```python
from build123d import *

# Parameters (mm, degrees)
SKETCH6_W                = 42.3
SKETCH6_H                = 42.3
SKETCH6_R                = 1.7
SKETCH6_R_2              = 13.5
BOSS_EXTRUDE4_DEPTH      = 6.35
SKETCH7_W                = 42.3
SKETCH7_H                = 6.35
BOSS_EXTRUDE5_DEPTH      = 6.35
SKETCH9_W                = 6.35
SKETCH9_H                = 6.35
BOSS_EXTRUDE7_DEPTH      = 20
BOSS_EXTRUDE9_DEPTH      = 12.7
BOSS_EXTRUDE9_DEPTH_BACK = 19.05
CUT_EXTRUDE3_DEPTH       = 62.003217128


with BuildPart() as part:
    # Sketch6 → Boss-Extrude4 (new body)
    with BuildSketch(Plane.XY):
        Rectangle(SKETCH6_W, SKETCH6_H)
        with Locations((-15.5, 15.5)):
            Circle(SKETCH6_R, mode=Mode.SUBTRACT)
        with Locations((15.5, 15.5)):
            Circle(SKETCH6_R, mode=Mode.SUBTRACT)
        with Locations((15.5, -15.5)):
            Circle(SKETCH6_R, mode=Mode.SUBTRACT)
        with Locations((-15.5, -15.5)):
            Circle(SKETCH6_R, mode=Mode.SUBTRACT)
        Circle(SKETCH6_R_2, mode=Mode.SUBTRACT)
    extrude(amount=BOSS_EXTRUDE4_DEPTH)

    # Sketch7 → Boss-Extrude5 (add)
    with BuildSketch(Plane(origin=(0, 21.15, 0), x_dir=(1, 0, 0), z_dir=(0, 1, 0))):
        with Locations((0, -3.175)):
            Rectangle(SKETCH7_W, SKETCH7_H)
    extrude(amount=BOSS_EXTRUDE5_DEPTH)

    # Sketch9 → Boss-Extrude7 (add)
    with BuildSketch(Plane(origin=(0, 27.5, 0), x_dir=(1, 0, 0), z_dir=(0, 1, 0))):
        with Locations((-17.975, -3.175)):
            Rectangle(SKETCH9_W, SKETCH9_H)
        with Locations((8.875, -3.175)):
            Rectangle(SKETCH9_W, SKETCH9_H)
    extrude(amount=BOSS_EXTRUDE7_DEPTH)

    # Sketch11 → Boss-Extrude9 (add, two sides: drawn at the far end of the back side and taken through both)
    with BuildSketch(Plane(origin=(0, 0, 0), x_dir=(-1, 0, 0), z_dir=(0, 0, -1)).offset(-BOSS_EXTRUDE9_DEPTH_BACK)):
        Polygon((-12.05, 47.5), (-12.05, 27.5), (-12.05, 21.15), (21.15, 21.15), (21.15, 47.5), (14.8, 47.5), (14.8, 27.5), (-5.7, 27.5), (-5.7, 47.5), align=None)
    extrude(amount=BOSS_EXTRUDE9_DEPTH + BOSS_EXTRUDE9_DEPTH_BACK)

    # Sketch12 → Cut-Extrude3 (cut, through all)
    with BuildSketch(Plane(origin=(12.05, 0, 0), x_dir=(0, 0, -1), z_dir=(1, 0, 0))):
        with BuildLine():
            ThreePointArc((2.5125, 37.5), (4.7625, 35.25), (7.0125, 37.5))
            Line((7.0125, 37.5), (2.5125, 37.5))
        make_face()
        with BuildLine():
            Line((2.5125, 37.5), (7.0125, 37.5))
            ThreePointArc((7.0125, 37.5), (4.7625, 39.75), (2.5125, 37.5))
        make_face()
        with BuildLine():
            ThreePointArc((-13.3625, 37.5), (-11.1125, 35.25), (-8.8625, 37.5))
            Line((-8.8625, 37.5), (-13.3625, 37.5))
        make_face()
        with BuildLine():
            Line((-13.3625, 37.5), (-8.8625, 37.5))
            ThreePointArc((-8.8625, 37.5), (-11.1125, 39.75), (-13.3625, 37.5))
        make_face()
    extrude(amount=-CUT_EXTRUDE3_DEPTH, mode=Mode.SUBTRACT)


solid = part.part
```
Work out the finished part from the listing and answer in its coordinate system (mm). A direction names the side the tool comes from. Give positions to 0.01 mm unless a question says otherwise; leave off trailing zeros. Loops run counter-clockwise (first coordinate to the right, second up) from the corner with the lowest first, then second, coordinate; pieces in that order, holes last. Notation, with made-up numbers: (2, 63.25) - (52, 63.25) arc R13 cw to (52, 81.25) - close; hole circle Ø8 at (-16, 51). An arc over 180 degrees is marked (long way). One line per question, with ' | ' between items.
(1) The part is cut by section C-C (z = 3). Write down the section's boundary in (x, y).
Recorded:
outline: (-21.15, -21.15) - (21.15, -21.15) - (21.15, 27.5) - (12.05, 27.5) - (12.05, 47.5) - (5.7, 47.5) - (5.7, 27.5) - (-14.8, 27.5) - (-14.8, 47.5) - (-21.15, 47.5) - close; hole circle Ø3.4 at (-15.5, -15.5); hole circle Ø3.4 at (-15.5, 15.5); hole circle Ø27 at (0, 0); hole circle Ø3.4 at (15.5, -15.5); hole circle Ø3.4 at (15.5, 15.5)
(2) Straight lines are drawn through the part: probe 1 along Y at (x, z) = (15.5, 5); probe 2 along X at (y, z) = (31, -5); probe 3 along Y at (x, z) = (-15, 2). For each, find the intervals that lie inside material, in ascending order.
Recorded:
probe 1: y = -21.15 to -17.2, -13.8 to 13.8, 17.2 to 27.5 | probe 2: x = -21.15 to -14.8, 5.7 to 12.05 | probe 3: y = -21.15 to -17.12, -13.88 to 13.88, 17.12 to 47.5
(3) The mould has two halves that part along Y. Classify faces 3 (the face through (-14.7, 14, 3.1)), 4 (the face through (9, 47.5, 3)), 5 (the face through (5.7, 37, 3)): +Y half, -Y half, draft (parallel to the pull), parting line (faces both ways), or undercut.
Recorded:
face 3: undercut | face 4: +Y half | face 5: draft
(4) The part is cut by section A-A (x = -15.5). Write down the section's boundary in (y, z), then the cut area to 3 significant figures.
Recorded:
outline: (-21.15, 0) - (-17.2, 0) - (-17.2, 6.35) - (-21.15, 6.35) - close; (-13.8, 0) - (13.8, 0) - (13.8, 6.35) - (-13.8, 6.35) - close; (17.2, 0) - (21.15, 0) - (21.15, -12.7) - (47.5, -12.7) - (47.5, 19.05) - (21.15, 19.05) - (21.15, 6.35) - (17.2, 6.35) - close; hole circle Ø4.5 at (37.5, -4.76); hole circle Ø4.5 at (37.5, 11.11) | area: 1,030 mm²
(5) A tool of negligible diameter and unlimited length cuts with its end or side. For faces 1 (the face through (-14.8, 38, 3)), 2 (the face through (-17.93, 39.73, 11.41)), from which of +Z, -Z, +X, -X, +Y, -Y can it reach the whole face along a straight path? Write none if from no direction.
Recorded:
face 1: +Z, -Z, +Y | face 2: +X, -X
(6) Each of these flat-tipped pins is pushed along its axis until it touches: pin 1 Ø4 at (y, z) = (37.5, -4.76) entering from +X; pin 2 Ø12 at (x, z) = (1.5, 9) entering from -Y; pin 3 Ø21 at (x, y) = (-2, -3.5) entering from +Z; pin 4 Ø16 at (y, z) = (40, 1) entering from +X. Where does it stop, or does it pass through?
Recorded:
pin 1: passes through | pin 2: stops at y = -21.15 | pin 3: stops at z = 6.35 | pin 4: stops at x = 12.05
(7) The part is cut by section B-B (y = 37.5). Write down the section's boundary in (x, z).
Recorded:
outline: (-21.15, -12.7) - (-14.8, -12.7) - (-14.8, -7.01) - (-21.15, -7.01) - close; (-21.15, -2.51) - (-14.8, -2.51) - (-14.8, 8.86) - (-21.15, 8.86) - close; (-21.15, 13.36) - (-14.8, 13.36) - (-14.8, 19.05) - (-21.15, 19.05) - close; (5.7, -12.7) - (12.05, -12.7) - (12.05, -7.01) - (5.7, -7.01) - close; (5.7, -2.51) - (12.05, -2.51) - (12.05, 8.86) - (5.7, 8.86) - close; (5.7, 13.36) - (12.05, 13.36) - (12.05, 19.05) - (5.7, 19.05) - close
(8) The part is cut by section D-D (x = 0). Write down the section's boundary in (y, z).
Recorded:
outline: (-21.15, 0) - (-13.5, 0) - (-13.5, 6.35) - (-21.15, 6.35) - close; (13.5, 0) - (21.15, 0) - (21.15, -12.7) - (27.5, -12.7) - (27.5, 19.05) - (21.15, 19.05) - (21.15, 6.35) - (13.5, 6.35) - close
